Read the model definition and answer for the solid it produces. Units are mm, in the model's axes. A direction names the side the tool comes from. Round coordinates to 2 decimals unless told otherwise and drop trailing zeros. Order: outer loops, then holes, each group sorted by start corner. A loop starts at its lowest first (then second) coordinate and runs counter-clockwise, first axis right, second up.
from build123d import *

# Parameters (mm, degrees)
F0_R     = 1.5
F0_W     = 41
F0_H     = 13
F0_W_2   = 10
F0_H_2   = 4
F7_DEPTH = 2
F4_W     = 41
F4_H     = 27
F4_R     = 1.5
F8_DEPTH = 2
F6_W     = 10
F6_H     = 27
F5_W     = 10
F5_H     = 27
F9_DEPTH = 2
F10_R    = 2


with BuildPart() as f7:
    # F0 (on Top) → F7 (new body)
    with BuildSketch(Plane.XY):
        with BuildLine():
            Line((-13.645751, 17), (-17.5, 17))
            Line((-17.5, 17), (-20, 17))
            Line((-20, 17), (-30, 17))
            Line((-30, 17), (-30, 0))
            Line((-30, 0), (-20.5, 0))
            Line((-20.5, 0), (20.5, 0))
            Line((20.5, 0), (30, 0))
            Line((30, 0), (30, 17))
            Line((30, 17), (20, 17))
            Line((20, 17), (17.5, 17))
            Line((17.5, 17), (13.645751, 17))
            ThreePointArc((13.645751, 17), (14.645751, 15.645751), (15, 14))
            ThreePointArc((15, 14), (9.354249, 10.354249), (8.354249, 17))
            Line((8.354249, 17), (-8.354249, 17))
            ThreePointArc((-8.354249, 17), (-7.354249, 15.645751), (-7, 14))
            ThreePointArc((-7, 14), (-12.645751, 10.354249), (-13.645751, 17))
        make_face()
        with Locations((-18.5, 14)):
            Circle(F0_R, mode=Mode.SUBTRACT)
        with Locations((-11, 6.5)):
            Circle(F0_R, mode=Mode.SUBTRACT)
        with Locations((-3.5, 14)):
            Circle(F0_R, mode=Mode.SUBTRACT)
        with Locations((11, 6.5)):
            Circle(F0_R, mode=Mode.SUBTRACT)
        with Locations((3.5, 14)):
            Circle(F0_R, mode=Mode.SUBTRACT)
        with Locations((18.5, 14)):
            Circle(F0_R, mode=Mode.SUBTRACT)
        with BuildLine():
            Line((17.5, 25), (-17.5, 25))
            Line((-17.5, 25), (-17.5, 17))
            Line((-17.5, 17), (-13.645751, 17))
            ThreePointArc((-13.645751, 17), (-11, 18), (-8.354249, 17))
            Line((-8.354249, 17), (8.354249, 17))
            ThreePointArc((8.354249, 17), (11, 18), (13.645751, 17))
            Line((13.645751, 17), (17.5, 17))
            Line((17.5, 17), (17.5, 25))
        make_face()
        with Locations((-11, 21.5)):
            Circle(F0_R, mode=Mode.SUBTRACT)
        with Locations((11, 21.5)):
            Circle(F0_R, mode=Mode.SUBTRACT)
        with Locations((0, -6.5)):
            Rectangle(F0_W, F0_H)
        with Locations((25, 19)):
            Rectangle(F0_W_2, F0_H_2)
        with Locations((-25, 19)):
            Rectangle(F0_W_2, F0_H_2)
    extrude(amount=F7_DEPTH)

    # F4 (on face) → F8 (join)
    with BuildSketch(Plane(origin=(0, -13, 0), x_dir=(-1, 0, 0), z_dir=(0, 1, 0))):
        with Locations((0, 13.5)):
            Rectangle(F4_W, F4_H)
        with Locations((-10, 16.5)):
            Circle(F4_R, mode=Mode.SUBTRACT)
        with Locations((10, 16.5)):
            Circle(F4_R, mode=Mode.SUBTRACT)
    extrude(amount=F8_DEPTH)

    # F6 (on face) + F5 (on face) → F9 (join)
    with BuildSketch(Plane(origin=(0, 21, 0), x_dir=(-1, 0, 0), z_dir=(0, 1, 0))):
        with Locations((25, 13.5)):
            Rectangle(F6_W, F6_H)
        with BuildLine():
            ThreePointArc((24.5, 9), (22.5, 11), (24.5, 13))
            Line((24.5, 13), (25.5, 13))
            ThreePointArc((25.5, 13), (27.5, 11), (25.5, 9))
            Line((25.5, 9), (24.5, 9))
        make_face(mode=Mode.SUBTRACT)
        with BuildLine():
            ThreePointArc((24.5, 19), (22.5, 21), (24.5, 23))
            Line((24.5, 23), (25.5, 23))
            ThreePointArc((25.5, 23), (27.5, 21), (25.5, 19))
            Line((25.5, 19), (24.5, 19))
        make_face(mode=Mode.SUBTRACT)
    with BuildSketch(Plane(origin=(0, 21, 0), x_dir=(-1, 0, 0), z_dir=(0, 1, 0))):
        with Locations((-25, 13.5)):
            Rectangle(F5_W, F5_H)
        with BuildLine():
            ThreePointArc((-25.5, 9), (-27.5, 11), (-25.5, 13))
            Line((-25.5, 13), (-24.5, 13))
            ThreePointArc((-24.5, 13), (-22.5, 11), (-24.5, 9))
            Line((-24.5, 9), (-25.5, 9))
        make_face(mode=Mode.SUBTRACT)
        with BuildLine():
            ThreePointArc((-25.5, 19), (-27.5, 21), (-25.5, 23))
            Line((-25.5, 23), (-24.5, 23))
            ThreePointArc((-24.5, 23), (-22.5, 21), (-24.5, 19))
            Line((-24.5, 19), (-25.5, 19))
        make_face(mode=Mode.SUBTRACT)
    extrude(amount=-F9_DEPTH)

    # F10
    f10_edges = [f7.edges().sort_by_distance(p)[0] for p in [
        (0, -13, 0),
        (-30, 0, 1),
        (30, 0, 1),
        (25, 21, 0),
        (-25, 21, 0),
        (17.5, 25, 1),
        (-17.5, 25, 1),
        (30, 20, 27),
        (20, 20, 27),
        (-20, 20, 27),
        (-30, 20, 27),
        (-20.5, -12, 27),
        (20.5, -12, 27),
    ]]
    fillet(f10_edges, radius=F10_R)


solid = f7.part
Q1. A cutting plane is placed at D-D, the plane y = -1.5. Give the vertices of the cut face in (x, z), plus the area to 3 significant figures.
Outcome:
outline: (-20.5, 0) - (20.5, 0) - (20.5, 2) - (-20.5, 2) - close
area: 82.0 mm2
Q2. For faces 1 (the face through (9.8, 5.6, 1)), 2 (the face through (20.5, -11.3, 8.7)), 3 (the face through (-24, 0, 1)), 4 (the face through (27.5, 20, 21)), 5 (the face through (-20.6, 19.99, 26.43)), determine the directions among +Z, -Z, +X, -X, +Y, -Y from which every point of the face is accessible in a straight line to the end or side of a thin tool.
Outcome:
face 1: +Z, -Z
face 2: +Z, -Z, +X, -Y
face 3: +Z, -Z, -X, -Y
face 4: +Y, -Y
face 5: +Z, +Y
Q3. Straight lines are drawn through the part: probe 1 along Y at (x, z) = (11, 1.4); probe 2 along Z at (x, y) = (6.5, -1.5); probe 3 along Y at (x, z) = (23.5, 9). For each, find the intervals that lie inside material, in ascending order.
Outcome:
probe 1: y = -12.91 to 5, 8 to 10, 18 to 20, 23 to 25
probe 2: z = 0 to 2
probe 3: y = 19 to 21
Q4. A cutting plane is placed at A-A, the plane z = 11. Give the vertices of the cut face in (x, y).
Outcome:
outline: (-30, 19) - (-27.5, 19) - (-27.5, 21) - (-30, 21) - close; (-22.5, 19) - (-20, 19) - (-20, 21) - (-22.5, 21) - close; (-20.5, -13) - (20.5, -13) - (20.5, -11) - (-20.5, -11) - close; (20, 19) - (22.5, 19) - (22.5, 21) - (20, 21) - close; (27.5, 19) - (30, 19) - (30, 21) - (27.5, 21) - close
Q5. A cutting plane is placed at B-B, the plane x = -3.5. Give the vertices of the cut face in (y, z).
Outcome:
outline: (-13, 2) arc R2 ccw to (-11, 0) - (12.5, 0) - (12.5, 2) - (-11, 2) - (-11, 27) - (-13, 27) - close; (15.5, 0) - (25, 0) - (25, 2) - (15.5, 2) - close
Q6. A cutting plane is placed at C-C, the plane y = 11. Give the vertices of the cut face in (x, z), plus the area to 3 significant figures.
Outcome:
outline: (-30, 0) - (-13.65, 0) - (-13.65, 2) - (-30, 2) - close; (-8.35, 0) - (8.35, 0) - (8.35, 2) - (-8.35, 2) - close; (13.65, 0) - (30, 0) - (30, 2) - (13.65, 2) - close
area: 98.8 mm2
Q7. For a pull along X with two mould halves and no side action, classify faces 6 (the face through (19.9, -11.99, 26.43)), 7 (the face through (-25, 19, 15)), 8 (the face through (20.6, 19.99, 26.43)) as released by +X, released by -X, zero draft, split by the parting line, or undercut.
Outcome:
face 6: released by +X
face 7: zero draft
face 8: undercut
Q8. Flat-ended cylindrical pins translate along their axes: pin 1 (4 mm diameter, centred on x = 11, y = 21.5, fed in from +Z); pin 2 (3 mm diameter, centred on x = 27, z = 16, fed in from +Y); pin 3 (0.8 mm diameter, centred on x = -25, y = 20, fed in from -Z). Find the tip coordinate at first contact, or state that the pin passes through.
Outcome:
pin 1: stops at z = 2
pin 2: stops at y = 21
pin 3: stops at z = 0.09
